Here's how the part is built. I have some questions about the finished solid (model axes, mm). Face numbers are marked on the shaded views. A direction names the side the tool comes from. Coordinates: 2 decimals unless noted, no trailing zeros. Write each loop counter-clockwise with the first axis right and the second up, starting at its lowest first coordinate (ties: lowest second). Pieces come first, ordered by that corner, then holes.
Item 1: If I drill on line 1 (Y direction, x = 2.1, z = 0) (3 decimals); line 2 (Y direction, x = 1.75, z = 2); line 3 (X direction, y = 7.75, z = 4.25), over which ranges is the centre line in solid material (lowest first)?
Item 2: I'm going to push flat-ended pins straight in: pin 1 Ø1.5 at (x, y) = (4.5, -3.5) entering from -Z; pin 2 Ø7.5 at (y, z) = (0, 0) entering from +X; pin 3 Ø3 at (x, y) = (4.5, 1.5) entering from -Z; pin 4 Ø1.5 at (x, z) = (1.5, 5.5) entering from -Y. Where does each tip first touch, or does it pass through?
Item 3: If we section it at A-A (x = 1.5): Please give me the cut outline in (y, z) (3 decimals).
Item 4: For the marked faces 4 and 5, which set-ups out of +Z, -Z, +X, -X, +Y, -Y let a thin tool reach every point of the face, with its end or its side?
Item 5: We'd pull the mould along Z, two halves only. Please class the marked faces 1, 2 and 3: +Z half, -Z half, draft (parallel to the pull), parting line (faces both ways), or undercut.
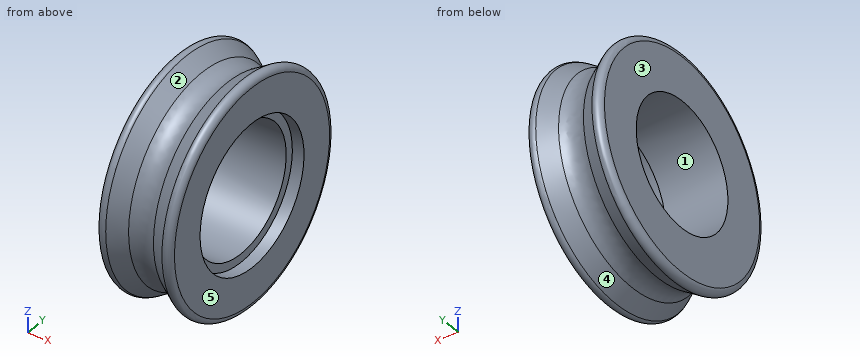
from build123d import *

# Parameters (mm, degrees)
FILLET1_R          = 0.5
FILLET2_R          = 2
SKETCH2_R          = 6.094107734
CUT_EXTRUDE1_DEPTH = 1
SKETCH3_R          = 5.375
CUT_EXTRUDE2_DEPTH = 6.35


with BuildPart() as part:
    # Sketch1 → Revolve1 (revolve)
    with BuildSketch(Plane.XY):
        Polygon((0, 0), (6.35, 0), (6.35, 10), (3.175, 8), (0, 10), align=None)
    revolve(axis=Axis((0, 0, 0), (1, 0, 0)))

    # Fillet1
    fillet1_edges = [part.edges().sort_by_distance(p)[0] for p in [
        (0, -10, 0),
        (6.35, -10, 0),
    ]]
    fillet(fillet1_edges, radius=FILLET1_R)

    # Fillet2
    fillet2_edges = [part.edges().sort_by_distance(p)[0] for p in [
        (3.175, -8, 0),
    ]]
    fillet(fillet2_edges, radius=FILLET2_R)

    # Sketch2 → Cut-Extrude1 (cut)
    with BuildSketch(Plane(origin=(6.35, 0, 0), x_dir=(0, 0, -1), z_dir=(1, 0, 0))):
        Circle(SKETCH2_R)
    extrude(amount=-CUT_EXTRUDE1_DEPTH, mode=Mode.SUBTRACT)

    # Sketch3 → Cut-Extrude2 (cut, through all)
    with BuildSketch(Plane(origin=(5.35, 0, 0), x_dir=(0, 0, -1), z_dir=(1, 0, 0))):
        Circle(SKETCH3_R)
    extrude(amount=-CUT_EXTRUDE2_DEPTH, mode=Mode.SUBTRACT)


solid = part.part
Answer list:
1. line 1: y = -8.677 to -5.375, 5.375 to 8.677
1. line 2: y = -8.67 to -4.99, 4.99 to 8.67
1. line 3: x = 0 to 1.84, 4.51 to 6.35
2. pin 1: stops at z = -8.7
2. pin 2: passes through
2. pin 3: stops at z = -9.56
2. pin 4: stops at y = -7.97
3. outline: circle Ø18.11 at (0, 0); hole circle Ø10.75 at (0, 0)
4. face 4: none
4. face 5: +Z, -Z, +X, +Y, -Y
5. face 1: undercut
5. face 2: parting line
5. face 3: draft
